```python
from build123d import *

# Parameters (mm, degrees)
SKETCH1_W           = 1600
SKETCH1_H           = 960
BOSS_EXTRUDE1_DEPTH = 20
SKETCH2_R           = 10
BOSS_EXTRUDE2_DEPTH = 20


with BuildPart() as part:
    # Sketch1 → Boss-Extrude1 (new body)
    with BuildSketch(Plane(origin=(0, 0, 0), x_dir=(1, 0, 0), z_dir=(0, 1, 0))):
        Rectangle(SKETCH1_W, SKETCH1_H)
    extrude(amount=-BOSS_EXTRUDE1_DEPTH)

    # Sketch2 → Boss-Extrude2 (add)
    with BuildSketch(Plane.XY.offset(480)):
        with BuildLine():
            Line((248, 0), (298, 0))
            Line((298, 0), (298, 100))
            ThreePointArc((298, 100), (273, 125), (248, 100))
            Line((248, 100), (248, 0))
        make_face()
        with Locations((273, 100)):
            Circle(SKETCH2_R, mode=Mode.SUBTRACT)
        with BuildLine():
            Line((680, 258.2), (680, 0))
            Line((680, 0), (730, 0))
            Line((730, 0), (730, 258.2))
            ThreePointArc((730, 258.2), (705, 283.2), (680, 258.2))
        make_face()
        with Locations((705, 258.2)):
            Circle(SKETCH2_R, mode=Mode.SUBTRACT)
    extrude(amount=-BOSS_EXTRUDE2_DEPTH)

    # Mirror1: part across plane


with BuildPart() as part_1:
    add(part.part)
    add(part.part.mirror(Plane.XY))


solid = part_1.part
```
Here's how the part is built. I have some questions about the finished solid (model axes, mm). Give positions to 0.01 mm unless a question says otherwise; leave off trailing zeros. Loops run counter-clockwise (first coordinate to the right, second up) from the corner with the lowest first, then second, coordinate; pieces in that order, holes last. Notation, with made-up numbers: (55, 54) -> (65, 54) arc R24 ccw to (65, 86) -> close; hole circle Ø3 at (41, 58). An arc over 180 degrees is marked (long way). Use one line per item in the form item = value. Start each with the question number.
1) Imagine slicing it at A-A (y = 34). Please give me the cut outline in (x, z), then the cut area to 3 significant figures.
2) Please list where these lines run through material, in increasing order: line 1 along Z through (x, y) = (713, 120); line 2 along Y through (x, z) = (705, 469.25); line 3 along Y through (x, z) = (273, -469.25).
3) For P1, Ø1, axis at x = 395.5, z = 281, coming from the +Y side; P2, Ø16, axis at x = 273, y = 100, coming from the -Z side; P3, Ø6, axis at y = 92.5, z = 465.5, coming from the +X side; P4, Ø6, axis at y = 188, z = 466, coming from the -X side, each with a flat end and sliding along its axis, tell me the tip position at first contact or that it passes through.
4) Imagine slicing it at C-C (x = -314). Please give me the cut outline in (y, z), then the cut area to 3 significant figures.
5) Thinking about a two-plate mould opening in Z: for faces 1 (the face through (273, 63, -460)), 2 (the face through (233, -2, -480)), 3 (the face through (-11, -20, -7)), 4 (the face through (233, -2, 480)), which applies, +Z half, -Z half, draft (parallel to the pull), parting line (faces both ways), or undercut?
6) Imagine slicing it at D-D (z = -85). Please give me the cut outline in (x, y), then the cut area to 3 significant figures.
7) Imagine slicing it at B-B (y = 147). Please give me the cut outline in (x, z).
Check values:
q1.outline = (248, -480) -> (298, -480) -> (298, -460) -> (248, -460) -> close; (248, 460) -> (298, 460) -> (298, 480) -> (248, 480) -> close; (680, -480) -> (730, -480) -> (730, -460) -> (680, -460) -> close; (680, 460) -> (730, 460) -> (730, 480) -> (680, 480) -> close
q1.area = 4,000 mm^2
q2.line_1 = -480 to -460, 460 to 480
q2.line_2 = -20 to 248.2, 268.2 to 283.2
q2.line_3 = -20 to 90, 110 to 125
q3.P1 = 0
q3.P2 = through
q3.P3 = 730
q3.P4 = 680
q4.outline = (-20, -480) -> (0, -480) -> (0, 480) -> (-20, 480) -> close
q4.area = 19,200 mm^2
q5.face_1 = undercut
q5.face_2 = -Z half
q5.face_3 = draft
q5.face_4 = +Z half
q6.outline = (-800, -20) -> (800, -20) -> (800, 0) -> (-800, 0) -> close
q6.area = 32,000 mm^2
q7.outline = (680, -480) -> (730, -480) -> (730, -460) -> (680, -460) -> close; (680, 460) -> (730, 460) -> (730, 480) -> (680, 480) -> close
